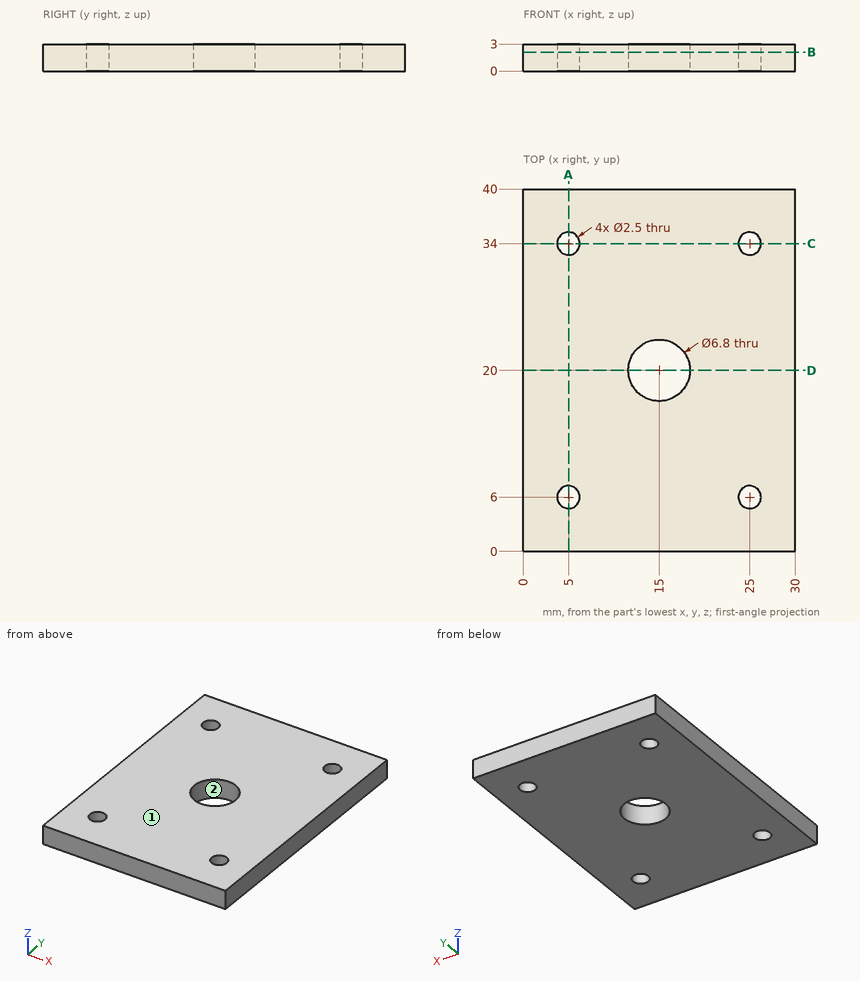
Check sheet for the drawn part. Datum: minimum x, y, z corner. Units: mm. Round coordinates to 2 decimals unless told otherwise and drop trailing zeros. Loops run counter-clockwise (first coordinate to the right, second up) from the corner with the lowest first, then second, coordinate; pieces in that order, holes last. Notation, with made-up numbers: (-40, 82) - (-7, 82) arc R17 cw to (-7, 109) - close; hole circle Ø11 at (21, 49). An arc over 180 degrees is marked (long way). Write each question's results on one line, items separated by ' | '. Start each with the question number.
Q1. Cross-section at B-B on z = 2.1. Enter the section's corners in (x, y).
Q2. Cross-section at A-A on x = 5. Enter the section's corners in (y, z).
Q3. Gauge pin test, flat end, axial feed: P1, Ø2, axis at x = 5, y = 34, coming from the +Z side. Record the tip position at first contact, or that the pin passes through.
Q4. Cross-section at D-D on y = 20. Enter the section's corners in (x, z), and give its area (3 significant figures).
Q5. Thickness scan on line 1 (Y direction, x = 5, z = 2.4); line 2 (X direction, y = 33, z = 2.85); line 3 (Y direction, x = 15, z = 1.5). Record the ranges inside material, lowest first. Write a range as [from, to].
Q6. Cross-section at C-C on y = 34. Enter the section's corners in (x, z), and give its area (3 significant figures).
Q7. Release check for a two-part mould opening along X. For the marked faces 1 and 2 record: +X half, -X half, draft (parallel to the pull), parting line (faces both ways), or undercut.
Answers below:
1) outline: (0, 0) - (30, 0) - (30, 40) - (0, 40) - close; hole circle Ø2.5 at (5, 6); hole circle Ø2.5 at (5, 34); hole circle Ø6.8 at (15, 20); hole circle Ø2.5 at (25, 6); hole circle Ø2.5 at (25, 34)
2) outline: (0, 0) - (4.75, 0) - (4.75, 3) - (0, 3) - close; (7.25, 0) - (32.75, 0) - (32.75, 3) - (7.25, 3) - close; (35.25, 0) - (40, 0) - (40, 3) - (35.25, 3) - close
3) P1: passes through
4) outline: (0, 0) - (11.6, 0) - (11.6, 3) - (0, 3) - close; (18.4, 0) - (30, 0) - (30, 3) - (18.4, 3) - close | area: 69.6 mm²
5) line 1: y = [0, 4.75], [7.25, 32.75], [35.25, 40] | line 2: x = [0, 4.25], [5.75, 24.25], [25.75, 30] | line 3: y = [0, 16.6], [23.4, 40]
6) outline: (0, 0) - (3.75, 0) - (3.75, 3) - (0, 3) - close; (6.25, 0) - (23.75, 0) - (23.75, 3) - (6.25, 3) - close; (26.25, 0) - (30, 0) - (30, 3) - (26.25, 3) - close | area: 75.0 mm²
7) face 1: draft | face 2: undercut
